Check sheet for the modelled part. Datum: model origin and axes. Units: mm. A direction names the side the tool comes from. Round coordinates to 2 decimals unless told otherwise and drop trailing zeros. Loops run counter-clockwise (first coordinate to the right, second up) from the corner with the lowest first, then second, coordinate; pieces in that order, holes last. Notation, with made-up numbers: M 89.25,5.25 L 114.25,5.25 A28 cw 114.25,36.25 Z; hole C 38.25,69 d7. An arc over 180 degrees is marked long. One line per question, with ' | ' between items. Start each with the question number.
(1) Thickness scan on probe 1 along X at (y, z) = (-13.5, 0.85). Record the ranges inside material, lowest first. Write a range as [from, to].
(2) Draft check along Y on faces 1 (the face through (63, 38.93, 2)), 2 (the face through (63, -7.153, 2)), 3 (the face through (-1, 12, 3)), 4 (the face through (-1, 80.213, 1)). Enter one of: +Y half, -Y half, draft (parallel to the pull), parting line (faces both ways), or undercut.
(3) Go/stop test with a flat-tipped pin: P1, Ø0.9, axis at y = 33.5, z = 2, coming from the +X side. Record where the tip stops, or that it passes through.
(4) Section check A-A (y = 32.5). Record the boundary of the cut face in (x, z), and give its area (3 significant figures).
(5) Tool access check on faces 5 (the face through (67.378, 12, 1)), 6 (the face through (59.378, 34, 2)). Record the directions out of +Z, -Z, +X, -X, +Y, -Y that give a thin tool (end or side, any length) a straight path to the whole face; none if there is none.
Autodesk Inventor part; units mm, degrees
ref_plane "YZ Plane" through (0, 0, 0) normal (1, 0, 0) x (0, 1, 0)
ref_plane "XZ Plane" through (0, 0, 0) normal (0, 1, 0) x (-1, 0, 0)
ref_plane "XY Plane" through (0, 0, 0) normal (0, 0, 1) x (1, 0, 0)
ref_plane "Work Plane1" through (0, 0, 0) normal (0, 0, 1) x (1, 0, 0)
sketch "Sketch1" plane through (0, 0, 0) normal (0, 0, 1) x (1, 0, 0)
  line L0 (67.3785, -57.1866) -> (-67.4215, -57.1866)
  line L1 (-67.4215, -57.1866) -> (-67.4215, 80.2134)
  line L2 (-67.4215, 80.2134) -> (67.3785, 80.2134)
  line L3 (67.3785, 80.2134) -> (67.3785, -57.1866)
  circle A0 centre (64.6972, 5.0885) radius 1
  circle A1 centre (-64.8231, 77.3114) radius 1
  circle A2 centre (64.7712, -54.4524) radius 1
  point P0 (0, 0)
  dimension "d0" = 2
  dimension "d1" = 2
  dimension "d4" = 2
  dimension "d11" = 137.4
  dimension "d12" = 134.8
extrude "Extrusion1" add sketch "Sketch1" along normal blind 3
sketch "Sketch2" plane through (0, 0, 3) normal (0, 0, 1) x (1, 0, 0)
  line L0 (67.3785, -57.1866) -> (67.3785, 80.2134)
  line L1 (67.3785, -16.1531) -> (59.3785, -16.1531)
  line L2 (59.3785, -16.1531) -> (59.3785, -7.1531)
  line L3 (59.3785, -7.1531) -> (67.3785, -7.1531)
  line L4 (67.3785, -7.1531) -> (67.3785, -16.1531)
  line L5 (67.3785, 29.9305) -> (59.3785, 29.9305)
  line L6 (59.3785, 29.9305) -> (59.3785, 38.9305)
  line L7 (59.3785, 38.9305) -> (67.3785, 38.9305)
  line L8 (67.3785, 38.9305) -> (67.3785, 29.9305)
  point P0 (0, 0)
  dimension "d5" = 8
  dimension "d6" = 9
  dimension "d7" = 8
  dimension "d8" = 9
extrude "Extrusion2" cut sketch "Sketch2" against normal through all
properties part number "CoverPSU"
The answers:
1) probe 1: [-67.42, 59.38]
2) face 1: undercut | face 2: undercut | face 3: draft | face 4: +Y half
3) P1: x = 59.38
4) outline: M -67.42,0 L 59.38,0 L 59.38,3 L -67.42,3 Z | area: 380 mm²
5) face 5: +Z, -Z, +X, +Y, -Y | face 6: +Z, -Z, +X
